from build123d import *

# Parameters (mm, degrees)
SKETCH2_R           = 1.6
BOSS_EXTRUDE1_DEPTH = 10
BOSS_EXTRUDE2_DEPTH = 46
CUT_EXTRUDE1_START  = -6
SKETCH5_W           = 5
SKETCH5_H           = 13
CUT_EXTRUDE1_DEPTH  = 6
FILLET1_R           = 1
FILLET2_R           = 0.5
FILLET3_R           = 1


with BuildPart() as part:
    # Sketch2 → Boss-Extrude1 (new body)
    with BuildSketch(Plane(origin=(0, 0, 0), x_dir=(1, 0, 0), z_dir=(0, 1, 0))):
        with BuildLine():
            ThreePointArc((-10, 0), (-7.22497216, 8.366600265), (0, 13.416407865))
            ThreePointArc((0, 13.416407865), (1.97882585, 13.853333716), (4, 14))
            Line((4, 14), (16, 14))
            Line((16, 14), (16, 23))
            Line((16, 23), (-16, 23))
            Line((-16, 23), (-16, -23))
            Line((-16, -23), (16, -23))
            Line((16, -23), (16, -14))
            Line((16, -14), (4, -14))
            ThreePointArc((4, -14), (-5.899494937, -9.899494937), (-10, 0))
        make_face()
        with Locations(Location((-12, -19, 0), (0, 0, 270))):
            Circle(SKETCH2_R, mode=Mode.SUBTRACT)
        with Locations(Location((0, -19, 0), (0, 0, 270))):
            Circle(SKETCH2_R, mode=Mode.SUBTRACT)
        with Locations(Location((12, -19, 0), (0, 0, 270))):
            Circle(SKETCH2_R, mode=Mode.SUBTRACT)
        with BuildLine():
            ThreePointArc((-10.4, 19), (-10.86862915, 17.86862915), (-12, 17.4))
            ThreePointArc((-12, 17.4), (-13.13137085, 20.13137085), (-10.4, 19))
        make_face(mode=Mode.SUBTRACT)
        with BuildLine():
            ThreePointArc((1.6, 19), (1.13137085, 17.86862915), (0, 17.4))
            ThreePointArc((0, 17.4), (-1.13137085, 20.13137085), (1.6, 19))
        make_face(mode=Mode.SUBTRACT)
        with Locations(Location((12, 19, 0), (0, 0, 270))):
            Circle(SKETCH2_R, mode=Mode.SUBTRACT)
    extrude(amount=BOSS_EXTRUDE1_DEPTH)

    # Sketch4 → Boss-Extrude2 (add)
    with BuildSketch(Plane.XY.offset(23)):
        Polygon((-21, 0), (-16, 10), (-16, 0), align=None)
    extrude(amount=-BOSS_EXTRUDE2_DEPTH)

    # Sketch5 → Cut-Extrude1 (cut)
    with BuildSketch(Plane(origin=(0, 10, 0), x_dir=(1, 0, 0), z_dir=(0, 1, 0)).offset(CUT_EXTRUDE1_START)):
        with BuildLine():
            Line((-16, 0), (-10, 0))
            ThreePointArc((-10, 0), (-7.591939741, 7.850282354), (-1.196152423, 13))
            Line((-1.196152423, 13), (-16, 13))
            Line((-16, 13), (-16, 0))
        make_face()
        with Locations((-18.5, 6.5)):
            Rectangle(SKETCH5_W, SKETCH5_H)
        with BuildLine():
            ThreePointArc((-1.196152423, -13), (-7.591939741, -7.850282354), (-10, 0))
            Line((-10, 0), (-16, 0))
            Line((-16, 0), (-16, -13))
            Line((-16, -13), (-1.196152423, -13))
        make_face()
        with Locations((-18.5, -6.5)):
            Rectangle(SKETCH5_W, SKETCH5_H)
    extrude(amount=CUT_EXTRUDE1_DEPTH, mode=Mode.SUBTRACT)

    # Fillet1
    fillet1_edges = [part.edges().sort_by_distance(p)[0] for p in [
        (-8.598076211, 10, 13),
        (-10.098076211, 4, 13),
        (-10.098076211, 4, -13),
        (-8.598076211, 10, -13),
    ]]
    fillet(fillet1_edges, radius=FILLET1_R - 0.0001)  # a hair under: the kernel refuses the full size

    # Fillet2
    fillet2_edges = [part.edges().sort_by_distance(p)[0] for p in [
        (-21, 0, 0),
    ]]
    fillet(fillet2_edges, radius=FILLET2_R)

    # Fillet3
    fillet3_edges = [part.edges().sort_by_distance(p)[0] for p in [
        (16, 5, 14),
        (16, 5, 23),
        (16, 5, -23),
        (16, 5, -14),
    ]]
    fillet(fillet3_edges, radius=FILLET3_R)


solid = part.part
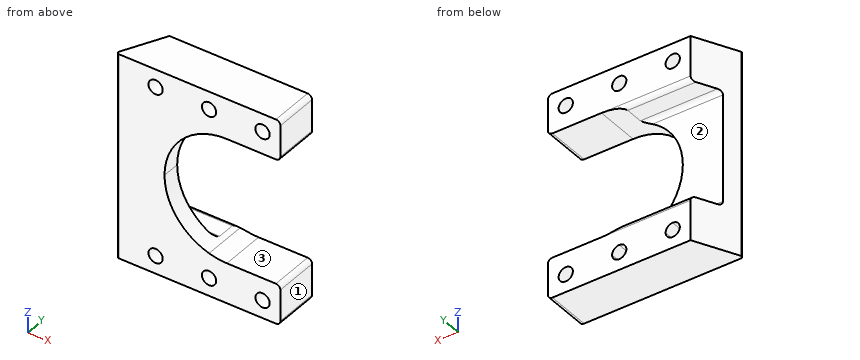
Model file for the job. Use its own axes, mm. Face numbers are marked on the shaded views. A direction names the side the tool comes from. Give positions to 0.01 mm unless a question says otherwise; leave off trailing zeros. Loops run counter-clockwise (first coordinate to the right, second up) from the corner with the lowest first, then second, coordinate; pieces in that order, holes last.
Item 1: Which spindle directions (+Z, -Z, +X, -X, +Y, -Y) get a long thin tool onto all of the face, cutting with end or side? Do the marked faces 1, 2 and 3. Say none if no direction does.
Check values:
face 1: +Z, -Z, +X, +Y, -Y
face 2: +X, -X, +Y
face 3: +X, +Y, -Y
Item 2: Slice it at D-D (z = 19). Write the cut outline in (x, y), plus the area to 3 significant figures.
Check values:
outline: (-20.64, 0.72) arc R0.5 ccw to (-20.19, 0) - (-13.6, 0) - (-13.6, 10) - (-16, 10) - close; (-10.4, 0) - (-1.6, 0) - (-1.6, 10) - (-10.4, 10) - close; (1.6, 0) - (10.4, 0) - (10.4, 10) - (1.6, 10) - close; (13.6, 0) - (16, 0) - (16, 10) - (13.6, 10) - close
area: 249 mm2
Item 3: Slice it at B-B (y = 3). Write the cut outline in (x, z).
Check values:
outline: (-19.5, -23) - (15, -23) arc R1 ccw to (16, -22) - (16, -15) arc R1 ccw to (15, -14) - (4, -14) arc R14 cw to (4, 14) - (15, 14) arc R1 ccw to (16, 15) - (16, 22) arc R1 ccw to (15, 23) - (-19.5, 23) - close; hole circle Ø3.2 at (-12, -19); hole circle Ø3.2 at (-12, 19); hole circle Ø3.2 at (0, -19); hole circle Ø3.2 at (0, 19); hole circle Ø3.2 at (12, -19); hole circle Ø3.2 at (12, 19)
Item 4: Drop flat-ended pins along their axis: P1, Ø3.5, axis at x = -12, z = -19, coming from the +Y side; P2, Ø12.5, axis at x = -8.5, z = 3, coming from the +Y side. Give the stop position or say it passes through.
Check values:
P1: stops at y = 10
P2: stops at y = 4
Item 5: Slice it at C-C (x = 12). Write the cut outline in (y, z), plus the area to 3 significant figures.
Check values:
outline: (0, -23) - (10, -23) - (10, -20.6) - (0, -20.6) - close; (0, -17.4) - (10, -17.4) - (10, -14) - (0, -14) - close; (0, 14) - (10, 14) - (10, 17.4) - (0, 17.4) - close; (0, 20.6) - (10, 20.6) - (10, 23) - (0, 23) - close
area: 116 mm2
Item 6: Slice it at A-A (y = 6). Write the cut outline in (x, z).
Check values:
outline: (-18, -23) - (15, -23) arc R1 ccw to (16, -22) - (16, -15) arc R1 ccw to (15, -14) - (4, -14) arc R14 cw to (-1.2, -13) - (-18, -13) - close; (-18, 13) - (-1.2, 13) arc R14 cw to (4, 14) - (15, 14) arc R1 ccw to (16, 15) - (16, 22) arc R1 ccw to (15, 23) - (-18, 23) - close; hole circle Ø3.2 at (-12, -19); hole circle Ø3.2 at (-12, 19); hole circle Ø3.2 at (0, -19); hole circle Ø3.2 at (0, 19); hole circle Ø3.2 at (12, -19); hole circle Ø3.2 at (12, 19)
Item 7: Drill centre lines: line 1 along Z through (x, y) = (-9, 9); line 2 along X through (y, z) = (8, -19.5); line 3 along X through (y, z) = (3.25, 19) (3 decimals). Where is each one in solid material? Low to high.
Check values:
line 1: z = -23 to -13, 13 to 23
line 2: x = -17 to -13.52, -10.48 to -1.52, 1.52 to 10.48, 13.52 to 16
line 3: x = -19.375 to -13.6, -10.4 to -1.6, 1.6 to 10.4, 13.6 to 16
